from build123d import *

# Parameters (mm, degrees)
SKETCH1_W           = 20
SKETCH1_H           = 20
SKETCH1_R           = 2.5
BOSS_EXTRUDE1_DEPTH = 1
SKETCH2_W           = 20
SKETCH2_H           = 20
SKETCH2_R           = 2.5
BOSS_EXTRUDE2_DEPTH = 1
BOSS_EXTRUDE3_DEPTH = 1
BOSS_EXTRUDE4_START = -19
BOSS_EXTRUDE4_DEPTH = 1
SKETCH5_W           = 5
SKETCH5_H           = 9
CUT_EXTRUDE1_DEPTH  = 24.685438565
SKETCH4_W           = 5
SKETCH4_H           = 10
CUT_EXTRUDE2_DEPTH  = 30.342801502


with BuildPart() as part:
    # Sketch1 → Boss-Extrude1 (new body)
    with BuildSketch(Plane(origin=(0, 0, 0), x_dir=(1, 0, 0), z_dir=(0, 1, 0))):
        Rectangle(SKETCH1_W, SKETCH1_H)
        with Locations(Location((0, 0, 0), (0, 0, 270))):
            Circle(SKETCH1_R, mode=Mode.SUBTRACT)
    extrude(amount=BOSS_EXTRUDE1_DEPTH)

    # Sketch2 → Boss-Extrude2 (add)
    with BuildSketch(Plane.XY.offset(10)):
        with Locations((0, 10)):
            Rectangle(SKETCH2_W, SKETCH2_H)
        with Locations((0, 10)):
            Circle(SKETCH2_R, mode=Mode.SUBTRACT)
    extrude(amount=-BOSS_EXTRUDE2_DEPTH)

    # Sketch3 → Boss-Extrude3 (add)
    with BuildSketch(Plane(origin=(10, 0, 0), x_dir=(0, 0, -1), z_dir=(1, 0, 0))):
        Polygon((-9, 10.5), (0.5, 1), (-9, 1), align=None)
    extrude(amount=-BOSS_EXTRUDE3_DEPTH)

    # Sketch3_2 → Boss-Extrude4 (add)
    with BuildSketch(Plane(origin=(10, 0, 0), x_dir=(0, 0, -1), z_dir=(1, 0, 0)).offset(BOSS_EXTRUDE4_START)):
        Polygon((-9, 10.5), (0.5, 1), (-9, 1), align=None)
    extrude(amount=-BOSS_EXTRUDE4_DEPTH)

    # Sketch5 → Cut-Extrude1 (cut, through all)
    with BuildSketch(Plane(origin=(0, 1, 0), x_dir=(1, 0, 0), z_dir=(0, 1, 0))):
        with Locations((0, -4.5)):
            Rectangle(SKETCH5_W, SKETCH5_H)
    extrude(amount=-CUT_EXTRUDE1_DEPTH, mode=Mode.SUBTRACT)

    # Sketch4 → Cut-Extrude2 (cut, through all)
    with BuildSketch(Plane(origin=(0, 0, 9), x_dir=(-1, 0, 0), z_dir=(0, 0, -1))):
        with Locations((0, 5)):
            Rectangle(SKETCH4_W, SKETCH4_H)
    extrude(amount=-CUT_EXTRUDE2_DEPTH, mode=Mode.SUBTRACT)


solid = part.part
Can you work these out from the model? Positions are in its coordinate system, mm. A direction names the side the tool comes from. Round coordinates to 2 decimals unless told otherwise and drop trailing zeros. Write each loop counter-clockwise with the first axis right and the second up, starting at its lowest first coordinate (ties: lowest second). Pieces come first, ordered by that corner, then holes. Notation, with made-up numbers: (72.25, 48) -> (101.25, 48) arc R11 cw to (101.25, 55) -> close; hole circle Ø10 at (-38, 85). An arc over 180 degrees is marked (long way). One line per question, with ' | ' between items. Start each with the question number.
1) If we mould it in two halves opening along X, with no side actions, what happens to faces 1 (the flat face through (10, 5, 5)), 2 (the cylindrical face through (0.1, 0.5, -2.5)), 3 (the flat face through (-2, 0, -2))? For each: released by +X, released by -X, zero draft, split by the parting line, or undercut.
2) Suppose I cut it at C-C on x = 0. Write out the boundary of the cut face in (y, z).
3) On a 3-axis mill with a long thin cutter (end or side, diameter ignored), from which of +Z, -Z, +X, -X, +Y, -Y can I reach the whole of each face in a straight line? I mean faces 4 (the flat face through (0, 1, -3)), 5 (the flat face through (-0.1, 20, 9.5)). Say none if no direction works.
4) Suppose I cut it at B-B on y = 2.75. Write out the boundary of the cut face in (x, z).
5) I'm going to push flat-ended pins straight in: P1, Ø1.5, axis at x = 0, z = 6.5, coming from the -Y side; P2, Ø5, axis at y = 8, z = 5, coming from the -X side; P3, Ø1, axis at x = -3.5, y = 12.5, coming from the -Z side; P4, Ø9.5, axis at x = -3.5, z = 0, coming from the +Y side. Where does each tip first touch, or does it pass through?
6) I need wall thicknesses on line 1 (X direction, y = 7.25, z = 7.5); line 2 (Z direction, x = 7.25, y = 2); line 3 (Y direction, x = -8.75, z = -1.25). Which ranges of each line are inside material? Lowest first, please. Write a range as [from, to].
7) Suppose I cut it at D-D on x = 3. Write out the boundary of the cut face in (y, z).
8) Suppose I cut it at A-A on z = 8.25. Write out the boundary of the cut face in (x, y), then the cut area to 3 significant figures.
Return value:
1) face 1: released by +X | face 2: undercut | face 3: zero draft
2) outline: (0, -10) -> (1, -10) -> (1, -2.5) -> (0, -2.5) -> close; (12.5, 9) -> (20, 9) -> (20, 10) -> (12.5, 10) -> close
3) face 4: -Z, +Y | face 5: +Z, -Z, +X, -X, +Y
4) outline: (-10, 1.25) -> (-9, 1.25) -> (-9, 9) -> (-2.5, 9) -> (-2.5, 10) -> (-10, 10) -> close; (2.5, 9) -> (9, 9) -> (9, 1.25) -> (10, 1.25) -> (10, 10) -> (2.5, 10) -> close
5) P1: passes through | P2: stops at x = -10 | P3: stops at z = 9 | P4: stops at y = 1
6) line 1: x = [-10, -9], [9, 10] | line 2: z = [9, 10] | line 3: y = [0, 1]
7) outline: (0, -10) -> (1, -10) -> (1, 9) -> (20, 9) -> (20, 10) -> (0, 10) -> close
8) outline: (-10, 0) -> (-2.5, 0) -> (-2.5, 1) -> (-9, 1) -> (-9, 9.75) -> (-10, 9.75) -> close; (2.5, 0) -> (10, 0) -> (10, 9.75) -> (9, 9.75) -> (9, 1) -> (2.5, 1) -> close | area: 32.5 mm2
